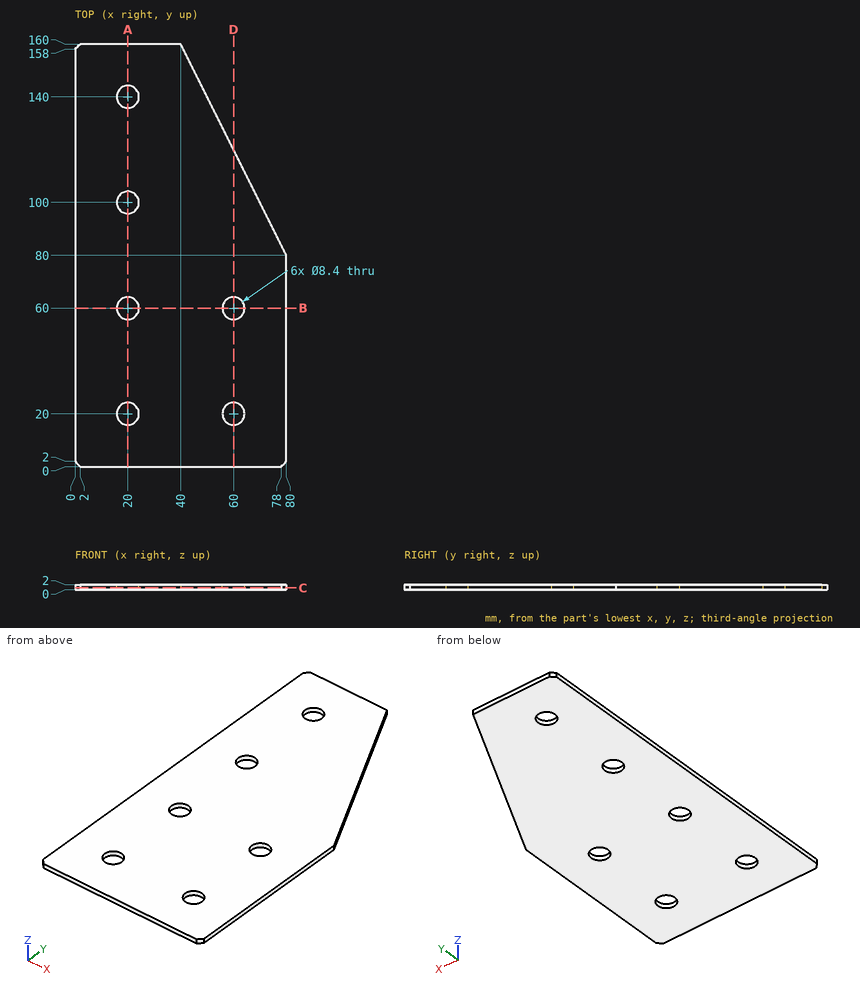
Verification items for this drawing (mm, ordinates from the low corner). Round coordinates to 2 decimals unless told otherwise and drop trailing zeros. Order: outer loops, then holes, each group sorted by start corner. A loop starts at its lowest first (then second) coordinate and runs counter-clockwise, first axis right, second up. Notation, with made-up numbers: (64, 19) -> (94, 19) arc R11 cw to (94, 39) -> close; hole circle Ø8 at (34.25, 83). An arc over 180 degrees is marked (long way). Use one line per item in the form item = value.
1. Cross-section at D-D, the plane x = 60. Enter the section's corners in (y, z), plus the area to 3 significant figures.
Working result:
outline = (0, 0) -> (15.8, 0) -> (15.8, 2) -> (0, 2) -> close; (24.2, 0) -> (55.8, 0) -> (55.8, 2) -> (24.2, 2) -> close; (64.2, 0) -> (120, 0) -> (120, 2) -> (64.2, 2) -> close
area = 206 mm^2
2. Cross-section at B-B, the plane y = 60. Enter the section's corners in (x, z), plus the area to 3 significant figures.
Working result:
outline = (0, 0) -> (15.8, 0) -> (15.8, 2) -> (0, 2) -> close; (24.2, 0) -> (55.8, 0) -> (55.8, 2) -> (24.2, 2) -> close; (64.2, 0) -> (80, 0) -> (80, 2) -> (64.2, 2) -> close
area = 126 mm^2
3. Cross-section at C-C, the plane z = 0.8. Enter the section's corners in (x, y).
Working result:
outline = (0, 2) -> (2, 0) -> (78, 0) -> (80, 2) -> (80, 80) -> (40, 160) -> (2, 160) -> (0, 158) -> close; hole circle Ø8.4 at (20, 20); hole circle Ø8.4 at (20, 60); hole circle Ø8.4 at (20, 100); hole circle Ø8.4 at (20, 140); hole circle Ø8.4 at (60, 20); hole circle Ø8.4 at (60, 60)
4. Cross-section at A-A, the plane x = 20. Enter the section's corners in (y, z), plus the area to 3 significant figures.
Working result:
outline = (0, 0) -> (15.8, 0) -> (15.8, 2) -> (0, 2) -> close; (24.2, 0) -> (55.8, 0) -> (55.8, 2) -> (24.2, 2) -> close; (64.2, 0) -> (95.8, 0) -> (95.8, 2) -> (64.2, 2) -> close; (104.2, 0) -> (135.8, 0) -> (135.8, 2) -> (104.2, 2) -> close; (144.2, 0) -> (160, 0) -> (160, 2) -> (144.2, 2) -> close
area = 253 mm^2
5. Scan lines: line 1 along Y through (x, z) = (20, 1.1); line 2 along Y through (x, z) = (63.5, 0.35); line 3 along Y through (x, z) = (58, 0.7). Record each from-to range of solid material in increasing order. Write a range as from..to.
Working result:
line_1 = 0..15.8, 24.2..55.8, 64.2..95.8, 104.2..135.8, 144.2..160
line_2 = 0..17.68, 22.32..57.68, 62.32..113
line_3 = 0..16.31, 23.69..56.31, 63.69..124
6. Go/stop test with a flat-tipped pin: pin 1 (6.5 mm diameter, centred on x = 60, y = 60, fed in from -Z). Record where the tip stops, or that it passes through.
Working result:
pin_1 = through
